from build123d import *

# Parameters (mm, degrees)
SKETCH1_W           = 33.5
SKETCH1_H           = 9.5
BOSS_EXTRUDE1_DEPTH = 10.8
CUT_EXTRUDE1_START  = -5
SKETCH2_R           = 6.05
CUT_EXTRUDE1_DEPTH  = 5
CUT_EXTRUDE2_START  = -3.8
SKETCH4_R           = 8.05
CUT_EXTRUDE2_DEPTH  = 3.8
SKETCH5_R           = 1.55
CUT_EXTRUDE3_DEPTH  = 10.5
SKETCH6_W           = 10
SKETCH6_H           = 10.8
BOSS_EXTRUDE2_DEPTH = 15
SKETCH7_R           = 1.55
CUT_EXTRUDE4_DEPTH  = 3
CUT_EXTRUDE5_DEPTH  = 2.75
FILLET1_R           = 2
BOSS_EXTRUDE3_DEPTH = 5
BOSS_EXTRUDE4_REACH = 10.8


with BuildPart() as part:
    # Sketch1 → Boss-Extrude1 (new body)
    with BuildSketch(Plane.XY):
        with Locations((4.4, -4.75)):
            Rectangle(SKETCH1_W, SKETCH1_H)
    extrude(amount=BOSS_EXTRUDE1_DEPTH)

    # Sketch2 → Cut-Extrude1 (cut)
    with BuildSketch(Plane.XY.offset(10.8).offset(CUT_EXTRUDE1_START)):
        with Locations((4.4, -12.5)):
            Circle(SKETCH2_R)
    extrude(amount=CUT_EXTRUDE1_DEPTH, mode=Mode.SUBTRACT)

    # Sketch4 → Cut-Extrude2 (cut)
    with BuildSketch(Plane.XY.offset(5.8).offset(CUT_EXTRUDE2_START)):
        with Locations((4.4, -12.5)):
            Circle(SKETCH4_R)
    extrude(amount=CUT_EXTRUDE2_DEPTH, mode=Mode.SUBTRACT)

    # Sketch5 → Cut-Extrude3 (cut, through all)
    with BuildSketch(Plane(origin=(0, 0, 0), x_dir=(1, 0, 0), z_dir=(0, 1, 0))):
        with Locations((17.4, -5.4)):
            Circle(SKETCH5_R)
        with Locations((-8.6, -5.4)):
            Circle(SKETCH5_R)
    extrude(amount=-CUT_EXTRUDE3_DEPTH, mode=Mode.SUBTRACT)

    # Sketch6 → Boss-Extrude2 (add)
    with BuildSketch(Plane(origin=(0, 0, 0), x_dir=(1, 0, 0), z_dir=(0, 1, 0))):
        with Locations((4.4, -5.4)):
            Rectangle(SKETCH6_W, SKETCH6_H)
    extrude(amount=BOSS_EXTRUDE2_DEPTH)

    # Sketch7 → Cut-Extrude4 (cut)
    with BuildSketch(Plane(origin=(0, 15, 0), x_dir=(1, 0, 0), z_dir=(0, 1, 0))):
        with Locations((4.4, -5.4)):
            Circle(SKETCH7_R)
    extrude(amount=-CUT_EXTRUDE4_DEPTH, mode=Mode.SUBTRACT)

    # Sketch8 → Cut-Extrude5 (cut)
    with BuildSketch(Plane(origin=(0, 12, 0), x_dir=(1, 0, 0), z_dir=(0, 1, 0))):
        Polygon((1.55, 0), (7.25, 0), (7.25, -3.754551733), (7.25, -7.045448267), (4.4, -8.690896534), (1.55, -7.045448267), (1.55, -3.754551733), align=None)
    extrude(amount=-CUT_EXTRUDE5_DEPTH, mode=Mode.SUBTRACT)

    # Fillet1
    fillet1_edges = [part.edges().sort_by_distance(p)[0] for p in [
        (9.4, 0, 5.4),
        (-0.6, 0, 5.4),
    ]]
    fillet(fillet1_edges, radius=FILLET1_R)

    # Sketch9 → Boss-Extrude3 (add)
    with BuildSketch(Plane.XY.offset(10.8)):
        with BuildLine():
            Line((9.653808143, -9.5), (9.422200713, -9.5))
            ThreePointArc((9.422200713, -9.5), (4.4, -6.65), (-0.622200713, -9.5))
            Line((-0.622200713, -9.5), (-0.853808143, -9.5))
            ThreePointArc((-0.853808143, -9.5), (4.4, -6.45), (9.653808143, -9.5))
        make_face()
    extrude(amount=-BOSS_EXTRUDE3_DEPTH)

    # Sketch10 → Boss-Extrude4 (add, up to next)
    with BuildSketch(Plane.XY.offset(2), mode=Mode.PRIVATE) as boss_extrude4_sk1:
        with BuildLine():
            Line((11.870107094, -9.5), (11.654136751, -9.5))
            ThreePointArc((11.654136751, -9.5), (4.4, -4.65), (-2.854136751, -9.5))
            Line((-2.854136751, -9.5), (-3.070107094, -9.5))
            ThreePointArc((-3.070107094, -9.5), (4.4, -4.45), (11.870107094, -9.5))
        make_face()
    boss_extrude4_tool1 = extrude(boss_extrude4_sk1.sketch, amount=BOSS_EXTRUDE4_REACH, mode=Mode.PRIVATE) - part.part
    add(boss_extrude4_tool1.solids().sort_by_distance((11.762122, -9.342294, 2))[0])


solid = part.part
Verification items for the finished model (mm, model axes). A direction names the side the tool comes from. Give positions to 0.01 mm unless a question says otherwise; leave off trailing zeros. Write each loop counter-clockwise with the first axis right and the second up, starting at its lowest first coordinate (ties: lowest second). Pieces come first, ordered by that corner, then holes. Notation, with made-up numbers: M 85,14 L 91,14 A22 cw 91,36 Z; hole C -11.5,-22 d3. An arc over 180 degrees is marked long. Use CSV: the item, a comma, the result in double quotes.
1) Access from +Z, -Z, +X, -X, +Y, -Y to the whole of each face (thin tool, end or side, straight path). Record for faces 1 (the face through (4.5, -6.5, 5.8)), 2 (the face through (-0.6, 8, 5)), 3 (the face through (4, 12, 3)).
Final values:
face 1,"-Y"
face 2,"+Z, -Z, -X, +Y"
face 3,"-Z"
2) Cross-section at C-C (z = 5.4). Enter the section's corners in (x, y), plus the area to 3 significant figures.
Final values:
outline,"M -12.35,-9.5 L -10.15,-9.5 L -10.15,0 L -12.35,0 Z; M -7.05,-9.5 L -2.85,-9.5 A7.85 cw 11.65,-9.5 L 15.85,-9.5 L 15.85,0 L 11.4,0 A2 cw 9.4,2 L 9.4,15 L 5.95,15 L 5.95,12 L 7.25,12 L 7.25,9.25 L 1.55,9.25 L 1.55,12 L 2.85,12 L 2.85,15 L -0.6,15 L -0.6,2 A2 cw -2.6,0 L -7.05,0 Z; M 18.95,-9.5 L 21.15,-9.5 L 21.15,0 L 18.95,0 Z"
area,"335 mm²"
3) Cross-section at A-A (x = 17.4). Enter the section's corners in (y, z), plus the area to 4 significant figures.
Final values:
outline,"M -9.5,0 L 0,0 L 0,3.85 L -9.5,3.85 Z; M -9.5,6.95 L 0,6.95 L 0,10.8 L -9.5,10.8 Z"
area,"73.15 mm²"
4) Go/stop test with flat-tipped pins: pin 1 Ø2.5 at (x, z) = (4.4, 5.4) entering from -Y; pin 2 Ø5 at (x, z) = (-6, 7) entering from +Y; pin 3 Ø2.5 at (x, z) = (17.4, 5.4) entering from -Y; pin 4 Ø2 at (y, z) = (11, 2) entering from +X. Record where each tip stops, or that it passes through.
Final values:
pin 1,"y = -6.77"
pin 2,"y = 0"
pin 3,"through"
pin 4,"x = 9.4"
5) Cross-section at D-D (z = 9.75). Enter the section's corners in (x, y).
Final values:
outline,"M -12.35,-9.5 L -0.62,-9.5 A5.85 cw 9.42,-9.5 L 21.15,-9.5 L 21.15,0 L 11.4,0 A2 cw 9.4,2 L 9.4,15 L -0.6,15 L -0.6,2 A2 cw -2.6,0 L -12.35,0 Z"
6) Release check for a two-part mould opening along Y. For faces 4 (the face through (1.55, 11, 3)), 5 (the face through (4.6, -9.5, 1.7)), 6 (the face through (4, -8, 2)), 7 (the face through (7.25, 11, 4)) record: released by +Y, released by -Y, zero draft, split by the parting line, or undercut.
Final values:
face 4,"undercut"
face 5,"released by -Y"
face 6,"zero draft"
face 7,"undercut"
7) Material ranges on line 1 along X through (y, z) = (-2.5, 5.4); line 2 along Z through (x, y) = (-8.6, -6.5); line 3 along X through (y, z) = (-6.5, 4.75), recorded low to high.
Final values:
line 1,"-12.35 to -10.15, -7.05 to 15.85, 18.95 to 21.15"
line 2,"0 to 3.85, 6.95 to 10.8"
line 3,"-12.35 to -10.01, -7.19 to -0.66, 9.46 to 15.99, 18.81 to 21.15"
8) Cross-section at B-B (y = 11). Enter the section's corners in (x, z), plus the area to 3 significant figures.
Final values:
outline,"M -0.6,0 L 1.55,0 L 1.55,7.05 L 4.4,8.69 L 7.25,7.05 L 7.25,0 L 9.4,0 L 9.4,10.8 L -0.6,10.8 Z"
area,"63.2 mm²"
